Print and shaded views of the part. All mm, measured from the part's lowest x, y and z. Coordinates: 2 decimals unless noted, no trailing zeros. Loops run counter-clockwise (first coordinate to the right, second up) from the corner with the lowest first, then second, coordinate; pieces in that order, holes last. Notation, with made-up numbers: (-4, 3.5) -> (18, 3.5) arc R7 ccw to (18, 16.5) -> close; hole circle Ø4 at (63, 59.25). An arc over 180 degrees is marked (long way). One line per item, written item: value. Start each with the question number.
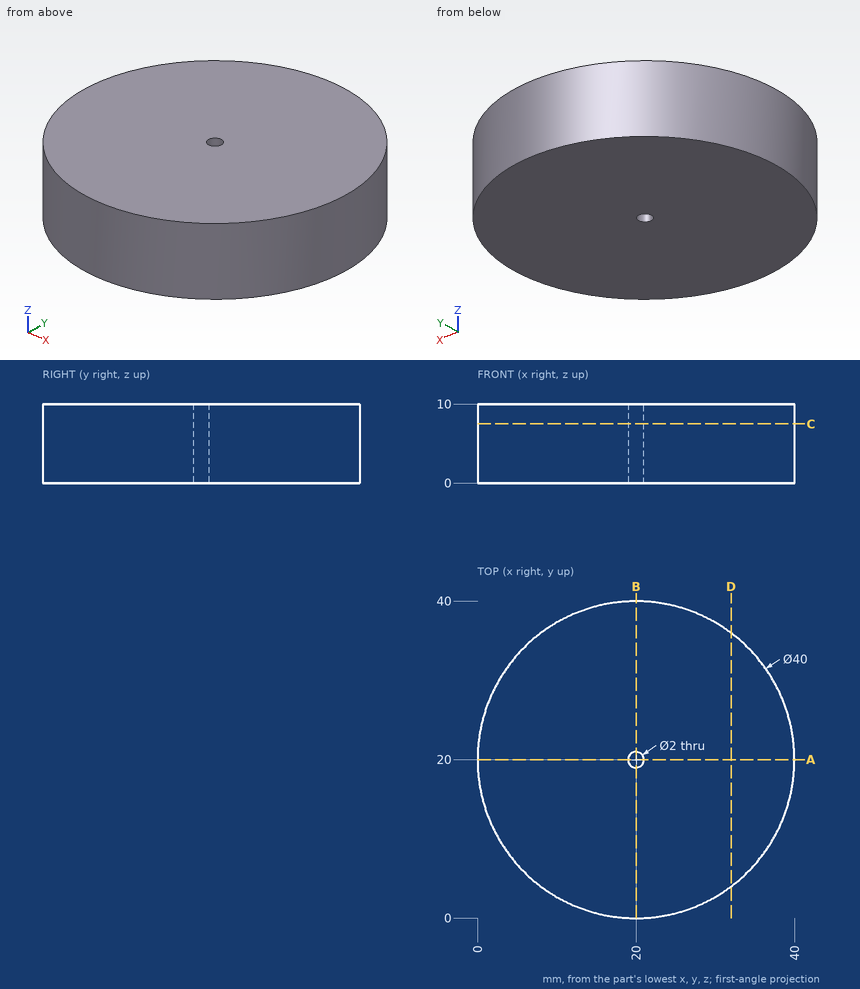
1) Slice it at A-A (y = 20). Give the cut face in (x, z), then the cut area to 3 significant figures.
2) Probe line 1 (Y direction, x = 20, z = 2.25); line 2 (X direction, y = 25.5, z = 3.25); line 3 (Y direction, x = 11, z = 2). List the from-to ranges inside material, lowest first. Write a range as from..to.
3) Slice it at D-D (x = 32). Give the cut face in (y, z).
4) Pin check, flat tips, straight feed: pin 1 Ø5 at (x, z) = (11.5, 5.5) entering from -Y; pin 2 Ø1.5 at (y, z) = (9, 3.5) entering from +X; pin 3 Ø2 at (x, z) = (33.5, 8.5) entering from -Y. Stop position of each tip, or through.
5) Slice it at C-C (z = 7.5). Give the cut face in (x, y), then the cut area to 3 significant figures.
Check sheet entries:
1. outline: (0, 0) -> (19, 0) -> (19, 10) -> (0, 10) -> close; (21, 0) -> (40, 0) -> (40, 10) -> (21, 10) -> close
1. area: 380 mm^2
2. line 1: y = 0..19, 21..40
2. line 2: x = 0.77..39.23
2. line 3: y = 2.14..37.86
3. outline: (4, 0) -> (36, 0) -> (36, 10) -> (4, 10) -> close
4. pin 1: stops at y = 0.92
4. pin 2: stops at x = 37.17
4. pin 3: stops at y = 4.39
5. outline: circle Ø40 at (20, 20); hole circle Ø2 at (20, 20)
5. area: 1,250 mm^2
